Geometry: final body of the model. Coordinates: model frame, mm. Round coordinates to 2 decimals unless told otherwise and drop trailing zeros. Loops run counter-clockwise (first coordinate to the right, second up) from the corner with the lowest first, then second, coordinate; pieces in that order, holes last. Notation, with made-up numbers: (39.25, 15) - (44.25, 15) arc R21 ccw to (44.25, 40) - close; hole circle Ø10 at (71.25, -15). An arc over 180 degrees is marked (long way). Use CSV: the item, a comma, the result in double quotes.
Autodesk Inventor part; units mm, degrees
ref_plane "YZ Plane" through (0, 0, 0) normal (1, 0, 0) x (0, 1, 0)
ref_plane "XZ Plane" through (0, 0, 0) normal (0, 1, 0) x (-1, 0, 0)
ref_plane "XY Plane" through (0, 0, 0) normal (0, 0, 1) x (1, 0, 0)
sketch "Block1" plane through (0, 0, 0) normal (0, 0, 1) x (1, 0, 0)
  circle A0 centre (47.0944, 34.7657) radius 2.1844
  circle A1 centre (-55.5339, 40.771) radius 2.0955
  arc A2 (-59.2675, 45.9074) -> (-52.0623, 35.454) centre (-55.5339, 40.771) ccw
  arc A3 (43.0264, 29.8899) -> (53.4444, 34.7657) centre (47.0944, 34.7657) ccw
  arc A4 (43.0264, 29.8899) -> (-52.0623, 35.454) centre (-8.279, -31.6038) ccw
  circle A5 centre (47.0944, 72.8657) radius 2.1844
  arc A6 (53.4444, 72.8657) -> (47.2364, 79.2141) centre (47.0944, 72.8657) ccw
  arc A7 (47.2364, 79.2141) -> (-59.2675, 45.9074) centre (43.3348, -95.2454) ccw
  circle A8 centre (-34.925, 52.3875) radius 2.0955
  point P0 (37.587, 35.3505)
  dimension "d2" = 12.7
  dimension "d3" = 12.7
  dimension "d4" = 12.7
  dimension "d9" = 4.191
sketch "Sketch1" plane through (0, 0, 0) normal (0, 0, 1) x (1, 0, 0)
  arc A0 (3.787, 33.0028) -> (0.142, 44.4484) centre (0, 38.1) ccw
  arc A1 (-4.068, -4.8758) -> (3.787, 5.0972) centre (0, 0) ccw
  arc A2 (3.787, 33.0028) -> (3.787, 5.0972) centre (14.1532, 19.05) ccw
  circle A3 centre (0, 0) radius 2.1844
  circle A4 centre (-102.6283, 6.0053) radius 2.0955
  arc A5 (-106.3619, 11.1417) -> (-99.1567, 0.6883) centre (-102.6283, 6.0053) ccw
  arc A6 (-4.068, -4.8758) -> (6.35, 0) centre (0, 0) ccw
  arc A7 (-4.068, -4.8758) -> (-99.1567, 0.6883) centre (-55.3735, -66.3695) ccw
  circle A8 centre (0, 38.1) radius 2.1844
  arc A9 (6.35, 38.1) -> (0.142, 44.4484) centre (0, 38.1) ccw
  arc A10 (0.142, 44.4484) -> (-106.3619, 11.1417) centre (-3.7596, -130.0112) ccw
  circle A11 centre (-82.0194, 17.6218) radius 2.0955
  point P0 (6.35, 0)
  point P1 (6.35, 38.1)
extrude "Extrusion1" add sketch "Sketch1" along normal blind 1.5875
equation "\"BendRadius\" = Thickness"
equation "\"BendReliefWidth\" = Thickness"
equation "\"BendReliefDepth\" = 0.5 * Thickness"
equation "\"CornerReliefSize\" = 4 * Thickness"
equation "\"MinimumRemnant\" = 2 * Thickness"
equation "\"TransitionRadius\" = BendRadius"
equation "\"JacobiRadiusSize\" = BendRadius"
equation "\"GapSize\" = Thickness"
properties part number "triball_jig" material "Acetal Resin, White"
Item 1: Section A-A on y = 38.1. Return the cut outline in (x, z).
Final values:
outline,"(-50.56, 0) - (-2.18, 0) - (-2.18, 1.59) - (-50.56, 1.59) - close; (2.18, 0) - (6.35, 0) - (6.35, 1.59) - (2.18, 1.59) - close"
Item 2: Material intervals for line 1 (Y direction, x = 0, z = 0.4); line 2 (Y direction, x = -1, z = 1.35); line 3 (X direction, y = 5, z = 1.4), sorted ascending.
Final values:
line 1,"y = -6.35 to -2.18, 2.18 to 8.96, 29.14 to 35.92, 40.28 to 44.45"
line 2,"y = -6.27 to -1.94, 1.94 to 10.53, 27.57 to 36.16, 40.04 to 44.47"
line 3,"x = -108.9 to -104.47, -100.79 to -91.71, -19.04 to 3.91"
Item 3: Section C-C on x = -77. Return the cut outline in (y, z).
Final values:
outline,"(10.74, 0) - (28.38, 0) - (28.38, 1.59) - (10.74, 1.59) - close"
Item 4: Mould query, pull axis X, two halves, no side actions, for faces 1 (the flat face through (-39, 19, 0)), 2 (the cylindrical face through (5.075, -3.816, 0.783)), 3 (the cylindrical face through (2.084, -0.656, 0.783)), 4 (the cylindrical face through (-0.474, 40.232, 0.783)). Classes: released by +X, released by -X, zero draft, split by the parting line, or undercut.
Final values:
face 1,"zero draft"
face 2,"split by the parting line"
face 3,"undercut"
face 4,"undercut"
Item 5: Section B-B on z = 0.6. Return the cut outline in (x, y).
Final values:
outline,"(-106.36, 11.14) arc R6.35 ccw to (-99.16, 0.69) arc R80.09 cw to (-4.07, -4.88) arc R6.35 ccw (long way) to (3.79, 5.1) arc R17.38 cw to (3.79, 33) arc R6.35 ccw to (0.14, 44.45) arc R174.5 ccw to start; hole circle Ø4.19 at (-102.63, 6.01); hole circle Ø4.19 at (-82.02, 17.62); hole circle Ø4.37 at (0, 0); hole circle Ø4.37 at (0, 38.1)"
Item 6: Pin query (flat end, axial travel): P1, Ø2.5, axis at x = 0, y = 0, coming from the +Z side. Return the tip coordinate at first contact, or that it passes through.
Final values:
P1,"passes through"
Item 7: Section D-D on y = 27.5. Return the cut outline in (x, z).
Final values:
outline,"(-78.87, 0) - (-1.04, 0) - (-1.04, 1.59) - (-78.87, 1.59) - close"
